Autodesk Inventor part; units mm, degrees
ref_plane "Work Plane1" through (29, 0, 0) normal (0, -1, 0) x (1, 0, 0)
ref_plane "YZ Plane" through (0, 0, 0) normal (1, 0, 0) x (0, 1, 0)
ref_plane "XZ Plane" through (0, 0, 0) normal (0, 1, 0) x (-1, 0, 0)
sketch "Sketch1" plane through (0, 0, 0) normal (0, 0, 1) x (1, 0, 0)
  line L0 (-0.0931, 0) -> (12.7, 0)
  line L1 (12.7, 0) -> (12.7, 2.0828)
  line L2 (12.7, 2.0828) -> (1.5902, 2.0828)
  line L3 (1.5902, 2.0828) -> (0.0001, 2.0828)
  line L4 (0.0001, 2.0828) -> (0, 2.0828)
  line L5 (0, 2.0828) -> (0, 3.9624)
  line L6 (0, 3.9624) -> (-2.2098, 3.9624)
  line L7 (-2.2098, 3.9624) -> (-2.2098, 1.3785)
  line L8 (-2.2098, 1.3785) -> (-0.889, 1.3785)
  line L9 (-0.889, 1.3785) -> (-0.0931, 0)
  line L10 (-5.1918, 0) -> (15.682, 0)
  line L11 (0, -0.7925) -> (0, 4.7549)
  line L12 (1.5902, 2.0828) -> (0, 2.0828) construction
  dimension "d1" = 11.1098
  dimension "d2" = 1.5901
  dimension "d3" = 2.2098
  dimension "d4" = 1.3208
  dimension "d5" = 60
  dimension "d6" = 4.1656
  dimension "d7" = 4.1656
  dimension "d8" = 2.757
  dimension "d9" = 7.9248
  dimension "d26" = 12.7
revolve "Body" add sketch "Sketch1" angle 360 about axis through (-0.0931, 0, 0) along (1, 0, 0)
sketch "Sketch2" plane through (-2.2098, 0, 0) normal (-1, 0, 0) x (0, 0, 1)
  circle A0 centre (0, 0) radius 1.3785
  line L0 (0, -5.5474) -> (0, 5.5474)
  line L1 (-5.5474, 0) -> (5.5474, 0)
  line L2 (1.3785, 0) -> (0.6892, -1.1938)
  line L3 (0.6892, -1.1938) -> (-0.6892, -1.1938)
  line L4 (-0.6892, -1.1938) -> (-1.3785, 0)
  line L5 (-1.3785, 0) -> (-0.6892, 1.1938)
  line L6 (-0.6892, 1.1938) -> (0.6892, 1.1938)
  line L7 (0.6892, 1.1938) -> (1.3785, 0)
extrude "Slot" add sketch "Sketch2" against normal up to next contours L7 A0 | A0 L2 | L6 L0 A0 | A0 L0 L3 | L0 L6 A0 | A0 L3 L0 | L4 A0 | A0 L5
fillet "Fillet1" radius 1.9558 1 edges at (-2.2098, -3.9624, 0)
thread "Thread"
chamfer "Chamfer1" distance 0.4869 distance2 0.4869 1 edges at (12.7, -2.0828, 0) measured on face at (12.7, -0.1898, 0.4203)
ref_plane "Work Plane1" through (29, 0, 0) normal (0, -1, 0) x (1, 0, 0)
fillet "Fillet2" radius 0.1 1 edges at (0.0001, -2.0828, 0)
equation "\"d1\" = GEL"
equation "\"d3\" = KOH"
equation "\"d4\" = INTI"
equation "\"d6\" = GD"
equation "\"d7\" = BDM"
equation "\"d8\" = 1.1547 * SW"
equation "\"d9\" = KOD"
equation "\"d26\" = NLG"
equation "\"d30\" = R"
equation "\"d17\" = RR"
equation "\"d13\" = GEL"
equation "\"d15\" = -0.5 * SPD + 0.5 * GD"
equation "\"d16\" = GUL"
equation "\"GD\" = NND"
equation "\"NLG\" = 12.7"
equation "\"GEL\" = 11.10976"
equation "\"KOD\" = 7.9248"
equation "\"KOH\" = 2.2098"
equation "\"INTI\" = 1.3208"
equation "\"GAL\" = 1.59004"
equation "\"GUL\" = 0.48692"
equation "\"BDM\" = NND"
equation "\"SW\" = 2.3876"
equation "\"RR\" = 1.9558"
equation "\"SPD\" = 3.19176"
equation "\"R\" = 0.1"
equation "\"TOA\" = 30deg"
equation "\"GD1\" = SPD"
equation "\"THREADDIA\" = 4.1656"
equation "\"KOH1\" = 0.381"
equation "\"NND\" = 4.1656"
equation "\"E0\" = 2.75768"
properties part number "ANSI B18.3 - 8 - 32 x 1/2" material "Steel, Mild"
CAD build for the part. Positions are in the model's coordinates, mm. A direction names the side the tool comes from. Coordinates: 2 decimals unless noted, no trailing zeros. Write each loop counter-clockwise with the first axis right and the second up, starting at its lowest first coordinate (ties: lowest second). Pieces come first, ordered by that corner, then holes. Notation, with made-up numbers: (81, 67.5) - (115, 67.5) arc R19 ccw to (115, 101.5) - close; hole circle Ø6 at (32, 68.5). An arc over 180 degrees is marked (long way). Use a Markdown table: item, result. Add a question column.
Item 1: Band-saw the part on A-A, the plane x = 0.5. Give the cut face in (y, z), and give its area (3 significant figures).
Item 2: Flat gauge pins, fed straight in: pin 1 (1.1 mm diameter, centred on x = -1.5, z = 0, fed in from +Y); pin 2 (1.5 mm diameter, centred on x = -2, z = -0.5, fed in from -Y); pin 3 (1.5 mm diameter, centred on x = 5.5, z = 3, fed in from -Y). Where does each tip first touch, or does it go through?
Item 3: Mould opens along Z. For faces 1 (the face through (6.072, -1.535, -1.408)), 2 (the face through (-1.506, 0.605, 1.029)), 3 (the face through (12.7, 0, 0)), 4 (the face through (-1.51, 0.59, -1.04)) say: pulls with the +Z half, pulls with the -Z half, needs draft (parallel to the pull), parting line crosses it, or undercut.
Item 4: 3-axis set-ups, long thin cutter, end or side, ignore diameter. For faces 5 (the face through (-2.21, -1, -1)), 6 (the face through (-2, 1.194, 0)): which of +Z, -Z, +X, -X, +Y, -Y reach the whole face in a straight line?
Item 5: Drill centre lines: L1, parallel to Y at x = -1, z = 0.5; L2, parallel to Z at x = 9.25, y = 1.25; L3, parallel to Z at x = 1.25, y = 1.5. Where is each one in solid material? Low to high. Write a range as from..to.
Numbers:
| question | item | result |
|---|---|---|
| 1 | outline | circle Ø4.17 at (0, 0) |
| 1 | area | 13.6 mm2 |
| 2 | pin 1 | y = 3.83 |
| 2 | pin 2 | y = -3.66 |
| 2 | pin 3 | through |
| 3 | face 1 | parting line crosses it |
| 3 | face 2 | undercut |
| 3 | face 3 | needs draft |
| 3 | face 4 | undercut |
| 4 | face 5 | +Z, -Z, -X, +Y, -Y |
| 4 | face 6 | -X |
| 5 | L1 | -3.78..-1.19, 1.19..3.78 |
| 5 | L2 | -1.67..1.67 |
| 5 | L3 | -1.45..1.45 |
